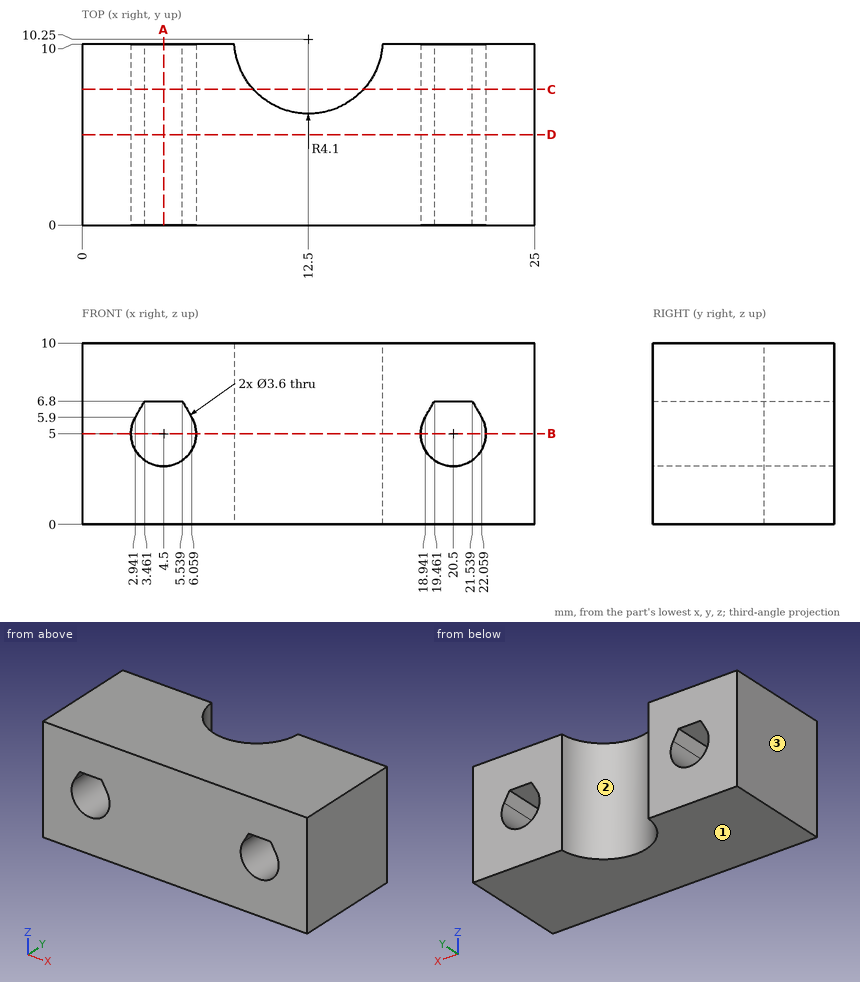
Source: three-view drawing plus pictorial views. Frame: mm from the lowest corner of the part. Coordinates: 2 decimals unless noted, no trailing zeros. Write each loop counter-clockwise with the first axis right and the second up, starting at its lowest first coordinate (ties: lowest second). Pieces come first, ordered by that corner, then holes. Notation, with made-up numbers: (43, 74) -> (99, 74) arc R16 ccw to (99, 99) -> close; hole circle Ø11 at (55, 70). An arc over 180 degrees is marked (long way). Write each question's results on one line, items separated by ' | '.
Item 1: Section query D-D on y = 5. Return loops of the section in (x, z), plus the area to 3 significant figures.
Conclusion:
outline: (0, 0) -> (25, 0) -> (25, 10) -> (0, 10) -> close; hole (2.94, 5.9) arc R1.8 ccw (long way) to (6.06, 5.9) -> (5.54, 6.8) -> (3.46, 6.8) -> close; hole (18.94, 5.9) arc R1.8 ccw (long way) to (22.06, 5.9) -> (21.54, 6.8) -> (19.46, 6.8) -> close | area: 229 mm^2
Item 2: Section query A-A on x = 4.5. Return loops of the section in (y, z), plus the area to 3 significant figures.
Conclusion:
outline: (0, 0) -> (10, 0) -> (10, 3.2) -> (0, 3.2) -> close; (0, 6.8) -> (10, 6.8) -> (10, 10) -> (0, 10) -> close | area: 64.0 mm^2
Item 3: Section query C-C on y = 7.5. Return loops of the section in (x, z), plus the area to 3 significant figures.
Conclusion:
outline: (0, 0) -> (9.46, 0) -> (9.46, 10) -> (0, 10) -> close; (15.54, 0) -> (25, 0) -> (25, 10) -> (15.54, 10) -> close; hole (2.94, 5.9) arc R1.8 ccw (long way) to (6.06, 5.9) -> (5.54, 6.8) -> (3.46, 6.8) -> close; hole (18.94, 5.9) arc R1.8 ccw (long way) to (22.06, 5.9) -> (21.54, 6.8) -> (19.46, 6.8) -> close | area: 168 mm^2
Item 4: Mould query, pull axis X, two halves, no side actions, for the marked faces 1, 2 and 3. Classes: +X half, -X half, draft (parallel to the pull), parting line (faces both ways), or undercut.
Conclusion:
face 1: draft | face 2: undercut | face 3: -X half
Item 5: Section query B-B on z = 5. Return loops of the section in (x, y).
Conclusion:
outline: (0, 0) -> (2.7, 0) -> (2.7, 10) -> (0, 10) -> close; (6.3, 0) -> (18.7, 0) -> (18.7, 10) -> (16.59, 10) arc R4.1 cw to (8.41, 10) -> (6.3, 10) -> close; (22.3, 0) -> (25, 0) -> (25, 10) -> (22.3, 10) -> close
Item 6: Material intervals for probe 1 along X at (y, z) = (4.25, 5); probe 2 along Z at (x, y) = (4.5, 5.75); probe 3 along X at (y, z) = (7.25, 5) (1 decimal), sorted ascending.
Conclusion:
probe 1: x = 0 to 2.7, 6.3 to 18.7, 22.3 to 25 | probe 2: z = 0 to 3.2, 6.8 to 10 | probe 3: x = 0 to 2.7, 6.3 to 9.7, 15.3 to 18.7, 22.3 to 25
